Can you work these out from the model? Positions are in its coordinate system, mm. A direction names the side the tool comes from. Round coordinates to 2 decimals unless told otherwise and drop trailing zeros. Write each loop counter-clockwise with the first axis right and the second up, starting at its lowest first coordinate (ties: lowest second). Pieces come first, ordered by that corner, then holes.
Q1. Please list where these lines run through material, in increasing order: line 1 along Y through (x, z) = (2.5, -9) (3 decimals); line 2 along Y through (x, z) = (-11.5, -1.25); line 3 along Z through (x, y) = (17, -11).
Q2. We'd pull the mould along X, two halves only. Please class faces 1 (the flat face through (30, -0.4, -4.4)), 2 (the flat face through (-30, -0.4, -5.8)), 3 (the cylindrical face through (2.52, -19.46, -8.87)), 4 (the flat face through (0, -5, -9.237)): +X half, -X half, draft (parallel to the pull), parting line (faces both ways), or undercut.
Q3. I'm going to push flat-ended pins straight in: pin 1 Ø0.6 at (x, y) = (0.5, -0.5) entering from +Z; pin 2 Ø0.6 at (y, z) = (-0.5, 2) entering from +X; pin 3 Ø10 at (y, z) = (-13, -2) entering from +X; pin 4 Ø2.5 at (x, y) = (2.9, -20.38) entering from +Z. Where does each tip first touch, or does it pass through?
Q4. If we section it at D-D (z = -5.75): Please give me the cut outline in (x, y).
Q5. If we section it at C-C (x = 18.5): Please give me the cut outline in (y, z).
Q6. If we section it at B-B (z = -0.5): Please give me the cut outline in (x, y), plus the area to 3 significant figures.
Q7. For faces 5 (the cylindrical face through (-4.249, -0.363, -3.708)), 6 (the cylindrical face through (-5.6, -8.9, -8.9)), 7 (the flat face through (0, -0.737, -5)), which set-ups out of +Z, -Z, +X, -X, +Y, -Y let a thin tool reach every point of the face, with its end or its side?
Q8. If we section it at A-A (y = -20.5): Please give me the cut outline in (x, z), plus the area to 3 significant figures.
from build123d import *

# Parameters (mm, degrees)
BASE_FLANGE1_DEPTH = 0.7366
EDGE_FLANGE1_DEPTH = 60
SKETCH10_R         = 1
CUT_EXTRUDE1_DEPTH = 10
SKETCH11_R         = 4.999999998
CUT_EXTRUDE2_DEPTH = 10
FILLET1_START      = -9.2366
FILLET1_DEPTH      = 0.7366
FILLET2_R          = 10
FILLET3_R          = 10
FILLET4_R          = 3
FILLET5_R          = 1
SKETCH14_R         = 5.07
SKETCH14_R_2       = 4.97
CUT_EXTRUDE4_DEPTH = 0.7366


with BuildPart() as part:
    # Base-Flange1: sheet metal written as solids
    # Sketch2 → Base-Flange1 (new body)
    with BuildSketch(Plane(origin=(0, 0, 0), x_dir=(1, 0, 0), z_dir=(0, 1, 0))):
        with BuildLine():
            Line((-2.36642583, 4.5), (7.36642583, 4.5))
            ThreePointArc((7.36642583, 4.5), (9.228643984, 3.728643984), (10, 1.86642583))
            Line((10, 1.86642583), (10, -4.86642583))
            ThreePointArc((10, -4.86642583), (10.771356016, -6.728643984), (12.63357417, -7.5))
            Line((12.63357417, -7.5), (30, -7.5))
            Line((30, -7.5), (30, 7.5))
            Line((30, 7.5), (-30, 7.5))
            Line((-30, 7.5), (-30, -7.5))
            Line((-30, -7.5), (-7.63357417, -7.5))
            ThreePointArc((-7.63357417, -7.5), (-5.771356016, -6.728643984), (-5, -4.86642583))
            Line((-5, -4.86642583), (-5, 1.86642583))
            ThreePointArc((-5, 1.86642583), (-4.228643984, 3.728643984), (-2.36642583, 4.5))
        make_face()
    extrude(amount=-BASE_FLANGE1_DEPTH)

    # Edge-Flange1: sheet metal written as solids
    # Edge-Flange1 section (on a plane across the edge) → Edge-Flange1 (add)
    with BuildSketch(Plane(origin=(-30, -0.7366, -8.5), x_dir=(0, 0, 1), z_dir=(1, 0, 0))):
        with BuildLine():
            Line((-0.7366, 0.7366), (-0.7366, 24.2634))
            Line((-0.7366, 24.2634), (0, 24.2634))
            Line((0, 24.2634), (0, 0.7366))
            ThreePointArc((0, 0.7366), (0.215745145, 0.215745145), (0.7366, 0))
            Line((0.7366, 0), (1, 0))
            Line((1, 0), (1, -0.7366))
            Line((1, -0.7366), (0.7366, -0.7366))
            ThreePointArc((0.7366, -0.7366), (-0.30510971, -0.30510971), (-0.7366, 0.7366))
        make_face()
    extrude(amount=EDGE_FLANGE1_DEPTH)

    # Sketch10 → Cut-Extrude1 (cut)
    with BuildSketch(Plane(origin=(0, 0, -9.2366), x_dir=(-1, 0, 0), z_dir=(0, 0, -1))):
        with Locations(Location((-9.590779371, -7.407129747, 0), (0, 0, 90))):
            Circle(SKETCH10_R)
        with Locations(Location((4.992621112, -8.103140058, 0), (0, 0, 90))):
            Circle(SKETCH10_R)
        with Locations(Location((-2.90184174, -20.384730194, 0), (0, 0, 90))):
            Circle(SKETCH10_R)
    extrude(amount=-CUT_EXTRUDE1_DEPTH, mode=Mode.SUBTRACT)

    # Sketch11 → Cut-Extrude2 (cut)
    with BuildSketch(Plane.XZ.offset(0.7366)):
        with Locations((22.255915642, 9.300009257)):
            Circle(SKETCH11_R)
    extrude(amount=-CUT_EXTRUDE2_DEPTH, mode=Mode.SUBTRACT)

    # Fillet1: read off the stored shape, not the designer's step
    # Fillet1 outline → Fillet1 (cut)
    with BuildSketch(Plane.XY.offset(FILLET1_START)):
        with BuildLine():
            ThreePointArc((30, -1.4732), (19.492381656, -18.390126122), (0.706695616, -25))
            Line((0.706695616, -25), (30, -25))
            Line((30, -25), (30, -1.4732))
        make_face()
        with BuildLine():
            ThreePointArc((-0.706695616, -25), (-19.492381656, -18.390126122), (-30, -1.4732))
            Line((-30, -1.4732), (-30, -25))
            Line((-30, -25), (-0.706695616, -25))
        make_face()
    extrude(amount=FILLET1_DEPTH, mode=Mode.SUBTRACT)

    # Fillet2
    fillet2_edges = [part.edges().sort_by_distance(p)[0] for p in [
        (-30, -0.3683, 7.5),
    ]]
    fillet(fillet2_edges, radius=FILLET2_R)

    # Fillet3
    # the kernel refuses this fillet: 10 mm, written as the material it takes off along each edge
    with BuildSketch(Plane(origin=(30, 18.045823122, 7.5), x_dir=(0, 0, -1), z_dir=(0, -1, 0))) as fillet3_piece_1:
        with BuildLine():
            CenterArc((7.218329249, -10), FILLET3_R, 90, 46.206018187)
            Line((0, -3.079326416), (-0.144366585, -2.940912944))
            ThreePointArc((-0.144366585, -2.940912944), (-0.2, -1.539663208), (-0.2, 0))
            Line((-0.2, 0), (0, 0.2))
            Line((0, 0.2), (7.218329249, 0.2))
            Line((7.218329249, 0.2), (7.218329249, 0))
        make_face()
    extrude(amount=36.828246244, mode=Mode.SUBTRACT)

    # Fillet4
    fillet4_edges = [part.edges().sort_by_distance(p)[0] for p in [
        (26.920673584, -0.3683, 7.5),
    ]]
    fillet(fillet4_edges, radius=FILLET4_R)

    # Fillet5
    fillet5_edges = [part.edges().sort_by_distance(p)[0] for p in [
        (17.5911577, -0.3683, 7.5),
    ]]
    fillet(fillet5_edges, radius=FILLET5_R)

    # Sketch14 → Cut-Extrude4 (cut)
    # profile 1 of 2: a face of its own
    with BuildSketch(Plane.XY.offset(-8.5)):
        with Locations((2.5, -11.965)):
            Circle(SKETCH14_R)
        with Locations((2.5, -11.965)):
            Circle(SKETCH14_R_2, mode=Mode.SUBTRACT)
    # profile 2 of 2: a face of its own
    with BuildSketch(Plane.XY.offset(-8.5)):
        with Locations((2.5, -11.965)):
            Circle(SKETCH14_R_2)
    extrude(amount=-CUT_EXTRUDE4_DEPTH, mode=Mode.SUBTRACT)


solid = part.part
A:
1. line 1: y = -24.946 to -21.3, -19.469 to -17.035, -6.895 to -0.672
1. line 2: y = -0.74 to 0
1. line 3: z = -9.24 to -8.5
2. face 1: +X half
2. face 2: -X half
2. face 3: undercut
2. face 4: draft
3. pin 1: stops at z = -4.5
3. pin 2: stops at x = 29.9
3. pin 3: passes through
3. pin 4: stops at z = -8.5
4. outline: (-30, -0.74) - (30, -0.74) - (30, 0) - (-30, 0) - close
5. outline: (-19.15, -9.24) - (-1.47, -9.24) arc R1.47 ccw to (0, -7.76) - (0, 6) - (-0.74, 6) - (-0.74, -7.76) arc R0.74 cw to (-1.47, -8.5) - (-19.15, -8.5) - close
6. outline: (-29.8, -0.74) - (-5, -0.74) - (-5, 0) - (-29.8, 0) - close; (10, -0.74) - (30, -0.74) - (30, 0) - (10, 0) - close
6. area: 33.0 mm2
7. face 5: +Z, +Y, -Y
7. face 6: +Z, -Z
7. face 7: +Z, +X, -X, -Y
8. outline: (-16.51, -9.24) - (1.91, -9.24) - (1.91, -8.5) - (-16.51, -8.5) - close; (3.9, -9.24) - (16.51, -9.24) - (16.51, -8.5) - (3.9, -8.5) - close
8. area: 22.9 mm2
